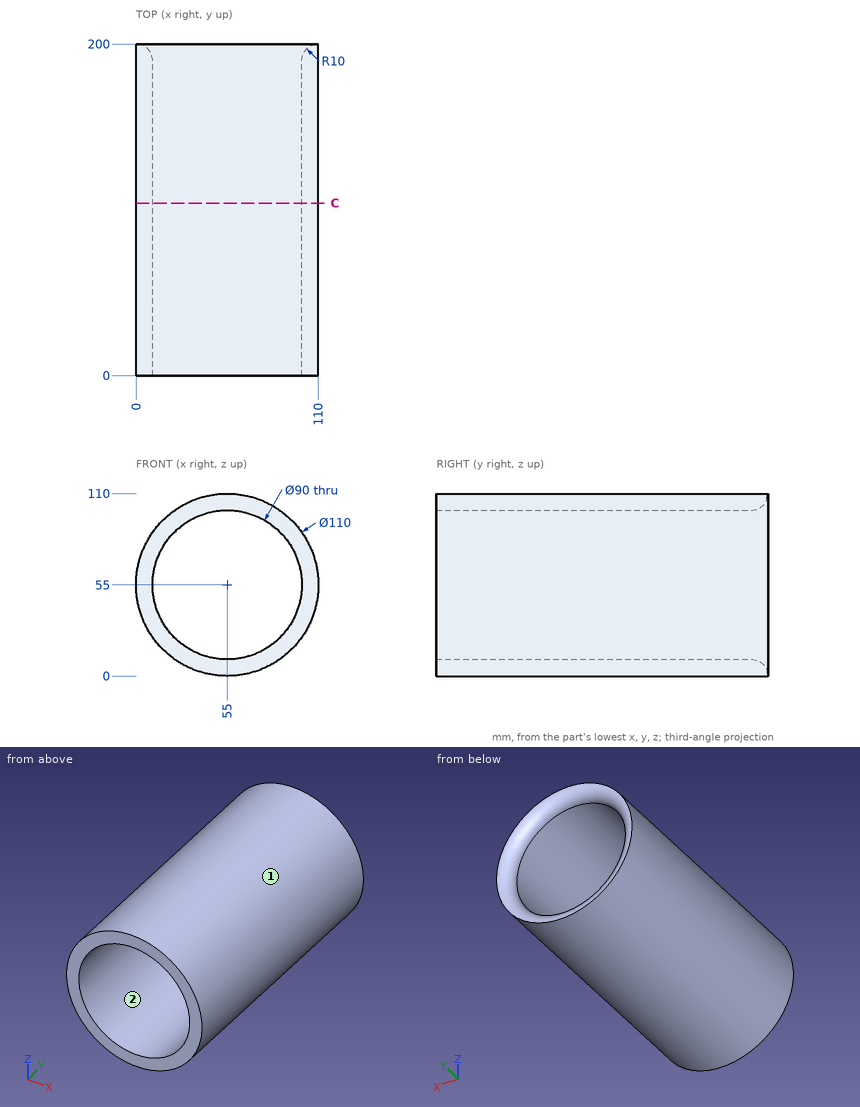
Can you work these out from the drawing? Everything is in mm from the part's minimum corner. Coordinates: 2 decimals unless noted, no trailing zeros. Loops run counter-clockwise (first coordinate to the right, second up) from the corner with the lowest first, then second, coordinate; pieces in that order, holes last.
1) I need wall thicknesses on probe 1 along X at (y, z) = (97, 55); probe 2 along Z at (x, y) = (38, 57) (1 decimal); probe 3 along X at (y, z) = (150.5, 42). Which ranges of each line are inside material? Lowest first, please.
2) For pin 1 (2 mm diameter, centred on y = 43, z = 50, fed in from +X); pin 2 (6 mm diameter, centred on x = 98, y = 151, fed in from -Z); pin 3 (3 mm diameter, centred on x = 41.5, y = 21.5, fed in from -Z) (3 decimals), each with a flat end and sliding along its axis, tell me the tip position at first contact or that it passes through.
3) Thinking about a two-plate mould opening in Z: for the marked faces 1 and 2, which applies, pulls with the +Z half, pulls with the -Z half, needs draft (parallel to the pull), parting line crosses it, or undercut?
4) Imagine slicing it at C-C on y = 104. List the corners of the cut face in (x, z) for me, plus the area to 3 significant figures.
Completed:
1. probe 1: x = 0 to 10, 100 to 110
1. probe 2: z = 2.7 to 13.3, 96.7 to 107.3
1. probe 3: x = 1.56 to 11.92, 98.08 to 108.44
2. pin 1: stops at x = 109.85
2. pin 2: stops at z = 17.25
2. pin 3: stops at z = 1.325
3. face 1: parting line crosses it
3. face 2: undercut
4. outline: circle Ø110 at (55, 55); hole circle Ø90 at (55, 55)
4. area: 3,140 mm2
